Source: CAD feature listing. Evaluate the final solid. Frame: model axes, mm. Face numbers are marked on the shaded views. A direction names the side the tool comes from. Give positions to 0.01 mm unless a question says otherwise; leave off trailing zeros. Write each loop counter-clockwise with the first axis right and the second up, starting at its lowest first coordinate (ties: lowest second). Pieces come first, ordered by that corner, then holes. Notation, with made-up numbers: (-8.75, 80.25) - (40.25, 80.25) arc R12 cw to (40.25, 97.25) - close; hole circle Ø1 at (41.25, 57.25). An arc over 180 degrees is marked (long way). Answer as a JSON object with one key per item and string values. Group by question number.
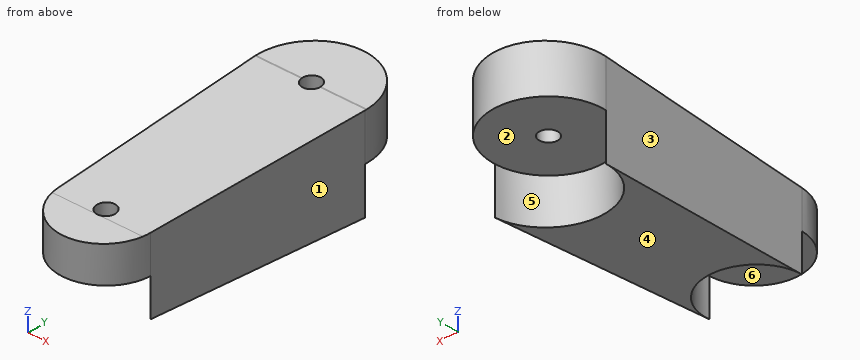
from build123d import *

# Parameters (mm, degrees)
F0_R     = 1.5875
F2_DEPTH = 12.7
F3_DEPTH = 12.7
F5_R     = 7.9375
F5_R_2   = 1.5875
F6_DEPTH = 25.4


with BuildPart() as f2:
    # F0 (on Top) → F2 (new body, symmetric)
    with BuildSketch(Plane.XY):
        with BuildLine():
            Line((7.930607, -38.430729), (9.516728, -0.396875))
            ThreePointArc((9.516728, -0.396875), (0, 9.525), (-9.516728, -0.396875))
            Line((-9.516728, -0.396875), (-7.930607, -38.430729))
            ThreePointArc((-7.930607, -38.430729), (0, -46.0375), (7.930607, -38.430729))
        make_face()
        with Locations((0, -38.1)):
            Circle(F0_R, mode=Mode.SUBTRACT)
        Circle(F0_R, mode=Mode.SUBTRACT)
    extrude(amount=F2_DEPTH, both=True)

    # F1 (on Right) → F3 (intersect, symmetric)
    with BuildSketch(Plane.YZ):
        Polygon((0, 7.943899), (-0.161479, 7.937414), (-39.6875, 6.35), (-46.0375, 6.094976), (-46.0375, -6.094976), (-39.6875, -6.35), (0, -7.943899), (9.525, -8.326434), (9.525, 8.326434), align=None)
    extrude(amount=F3_DEPTH, both=True, mode=Mode.INTERSECT)

    # F5 (on offset) → F6 (cut)
    with BuildSketch(Plane.XY):
        with BuildLine():
            ThreePointArc((-9.516728, -0.396875), (0, -9.525), (9.516728, -0.396875))
            ThreePointArc((9.516728, -0.396875), (9.522932, -0.198481), (9.525, 0))
            ThreePointArc((9.525, 0), (-0.198481, 9.522932), (-9.516728, -0.396875))
        make_face()
        with Locations((0, -38.1)):
            Circle(F5_R)
        with Locations((0, -38.1)):
            Circle(F5_R_2, mode=Mode.SUBTRACT)
    extrude(amount=-F6_DEPTH, mode=Mode.SUBTRACT)


solid = f2.part
Q1. Section D-D on x = 3.25. Return the cut outline in (y, z).
Q2. First-contact query: pin 1 Ø5 at (x, y) = (-2, -35) entering from -Z; pin 2 Ø5 at (x, y) = (-3, -9.5) entering from -Z; pin 3 Ø4 at (x, y) = (-7, -23) entering from +Z. Flat tips, straight axial feed; report the tip coordinate or a pass-through.
Q3. Draft query along X for the marked faces 1, 2 and 3. Return one class per face: released by +X, released by -X, zero draft, split by the parting line, or undercut.
Q4. Reachability of the marked faces 4, 5 and 6 from +Z, -Z, +X, -X, +Y, -Y: full face, straight path, thin tool, end or side. Return the list, or none.
Q5. Ray query, probe 1 along X at (y, z) = (-38.1, 1.5); probe 2 along Y at (x, z) = (0, 2.75) (1 decimal); probe 3 along X at (y, z) = (0, 6) (1 decimal). Return the intervals inside material, ascending. Write a range as [from, to].
Q6. Section A-A on z = 2.5. State how many separate pieces and enclosed holes the cut face has, then the cut area to 3 significant figures.
Q7. Section C-C on y = -34.5. Return the cut outline in (x, z).
Taken from the geometry:
{
 "1": {"outline": "(-45.34, 0) - (-30.86, 0) - (-30.86, -6.7) - (-8.95, -7.58) - (-8.95, 0) - (8.95, 0) - (8.95, 8.3) - (0, 7.94) - (-0.16, 7.94) - (-45.34, 6.12) - close"},
 "2": {"pin 1": "stops at z = 0", "pin 2": "stops at z = -7.62", "pin 3": "stops at z = 7.1"},
 "3": {"face 1": "released by +X", "face 2": "undercut", "face 3": "released by -X"},
 "4": {"face 4": "-Z, +X, -X, -Y", "face 5": "-Z, +Y", "face 6": "-Z, -Y"},
 "5": {"probe 1": "x = [-7.94, -1.59], [1.59, 7.94]", "probe 2": "y = [-46, -39.7], [-36.5, -1.6], [1.6, 9.5]", "probe 3": "x = [-9.5, -1.6], [1.6, 9.5]"},
 "6": {"separate pieces": "1", "enclosed holes": "2", "area": "892 mm²"},
 "7": {"outline": "(-8.09, -6.56) - (-7.07, -6.56) - (-7.07, 0) - (7.07, 0) - (7.07, -6.56) - (8.09, -6.56) - (8.09, 6.56) - (-8.09, 6.56) - close"}
}
